Model file for the job. Use its own axes, mm. A direction names the side the tool comes from. Coordinates: 2 decimals unless noted, no trailing zeros. Write each loop counter-clockwise with the first axis right and the second up, starting at its lowest first coordinate (ties: lowest second). Pieces come first, ordered by that corner, then holes. Notation, with made-up numbers: (73, 87) -> (80, 87) arc R11 ccw to (80, 104) -> close; hole circle Ø10 at (56.5, 38). An arc over 180 degrees is marked (long way). Write item = value, one per line. Start each with the question number.
from build123d import *

# Parameters (mm, degrees)
F1_DEPTH      = 30
F2_R          = 12.5
F3_DEPTH      = 25
F3_DEPTH_BACK = 25
F4_SIZE       = 2
F5_R          = 3
F6_DEPTH      = 44.501
F7_R          = 3
F8_DEPTH      = 25.001


with BuildPart() as f1:
    # F0 (on Front) → F1 (new body, symmetric)
    with BuildSketch(Plane.XZ):
        with BuildLine():
            Line((44.5, 0), (2.5, 0))
            ThreePointArc((2.5, 0), (0.732233047, -0.732233047), (0, -2.5))
            Line((0, -2.5), (0, -25))
            Line((0, -25), (4.5, -25))
            Line((4.5, -25), (4.5, -7))
            ThreePointArc((4.5, -7), (5.232233047, -5.232233047), (7, -4.5))
            Line((7, -4.5), (44.5, -4.5))
            Line((44.5, -4.5), (44.5, 0))
        make_face()
    extrude(amount=F1_DEPTH, both=True)

    # F2 (on Right) → F3 (join, two sides)
    with BuildSketch(Plane.YZ) as f3_sk:
        Circle(F2_R)
    extrude(amount=F3_DEPTH)
    extrude(f3_sk.sketch, amount=-F3_DEPTH_BACK)

    # F4
    f4_edges = [f1.edges().sort_by_distance(p)[0] for p in [
        (-25, -12.5, 0),
        (25, 0, 12.5),
    ]]
    chamfer(f4_edges, length=F4_SIZE)

    # F5 (on face) → F6 (cut, through all)
    with BuildSketch(Plane(origin=(0, 0, 0), x_dir=(0, -1, 0), z_dir=(-1, 0, 0))):
        with Locations((-20, -15)):
            Circle(F5_R)
        with Locations((20, -15)):
            Circle(F5_R)
    extrude(amount=-F6_DEPTH, mode=Mode.SUBTRACT)

    # F7 (on face) → F8 (cut, through all)
    with BuildSketch(Plane.XY):
        with Locations((34.5, 20)):
            Circle(F7_R)
        with Locations((34.5, -20)):
            Circle(F7_R)
    extrude(amount=-F8_DEPTH, mode=Mode.SUBTRACT)


solid = f1.part
(1) Drill centre lines: line 1 along Y through (x, z) = (34.5, -1.3); line 2 along Z through (x, y) = (3.25, -20); line 3 along X through (y, z) = (8, -19). Where is each one in solid material? Low to high.
(2) Saw through at D-D (y = 0). Give the cut face in (x, z).
(3) Mould opens along Z. For faces 1 (the face through (2.22, -19.35, -17.93)), 2 (the face through (4.5, 0, -16)), 3 (the face through (28, 0, 0)) say: released by +Z, released by -Z, zero draft, split by the parting line, or undercut.
(4) 3-axis set-ups, long thin cutter, end or side, ignore diameter. For faces 4 (the face through (5.213, 20.041, -5.252)), 5 (the face through (0, 0, -14)), 6 (the face through (25.5, -0.4, -4.5)): which of +Z, -Z, +X, -X, +Y, -Y reach the whole face in a straight line?
(5) Drop flat-ended pins along their axis: pin 1 Ø4 at (x, z) = (17, -5.5) entering from -Y; pin 2 Ø20 at (y, z) = (1.5, -19.5) entering from +X; pin 3 Ø5 at (x, y) = (34.5, -20) entering from -Z (1 decimal); pin 4 Ø8 at (y, z) = (6, -14.5) entering from -X. Give the stop position or say it passes through.
(6) Saw through at A-A (x = 34.5). Give the cut face in (y, z), then the cut area to 3 significant figures.
(7) Saw through at B-B (z = -15). Give the cut face in (x, y), then the cut area to 3 significant figures.
(8) Saw through at C-C (y = 20). Give the cut face in (x, z).
Returned:
q1.line_1 = -30 to -23, -17 to 17, 23 to 30
q1.line_2 = -25 to -18, -12 to 0
q1.line_3 = 0 to 4.5
q2.outline = (-25, -10.5) -> (-23, -12.5) -> (0, -12.5) -> (0, -25) -> (4.5, -25) -> (4.5, -12.5) -> (25, -12.5) -> (25, -4.5) -> (44.5, -4.5) -> (44.5, 0) -> (25, 0) -> (25, 10.5) -> (23, 12.5) -> (-23, 12.5) -> (-25, 10.5) -> close
q3.face_1 = undercut
q3.face_2 = zero draft
q3.face_3 = released by +Z
q4.face_4 = -Z, +X, +Y
q4.face_5 = -Z, -X
q4.face_6 = -Z, +X
q5.pin_1 = -30
q5.pin_2 = 25
q5.pin_3 = through
q5.pin_4 = -23.81
q6.outline = (-30, -4.5) -> (-23, -4.5) -> (-23, 0) -> (-30, 0) -> close; (-17, -4.5) -> (17, -4.5) -> (17, 0) -> (-17, 0) -> close; (23, -4.5) -> (30, -4.5) -> (30, 0) -> (23, 0) -> close
q6.area = 216 mm2
q7.outline = (0, -30) -> (4.5, -30) -> (4.5, -23) -> (0, -23) -> close; (0, -17) -> (4.5, -17) -> (4.5, 17) -> (0, 17) -> close; (0, 23) -> (4.5, 23) -> (4.5, 30) -> (0, 30) -> close
q7.area = 216 mm2
q8.outline = (0, -25) -> (4.5, -25) -> (4.5, -18) -> (0, -18) -> close; (0, -12) -> (4.5, -12) -> (4.5, -7) arc R2.5 cw to (7, -4.5) -> (31.5, -4.5) -> (31.5, 0) -> (2.5, 0) arc R2.5 ccw to (0, -2.5) -> close; (37.5, -4.5) -> (44.5, -4.5) -> (44.5, 0) -> (37.5, 0) -> close
